from build123d import *

# Parameters (mm, degrees)
F0_R     = 4.5
F1_DEPTH = 7.5


with BuildPart() as f1:
    # F0 (on Front) → F1 (new body, symmetric)
    with BuildSketch(Plane.XZ):
        with BuildLine():
            ThreePointArc((-29.920215, -2.18649), (1.093972, -29.980047), (30, 0))
            ThreePointArc((30, 0), (21.430167, 20.993997), (0.616805, 29.993659))
            ThreePointArc((0.616805, 29.993659), (-1.441951, 29.965326), (-3.493914, 29.795848))
            ThreePointArc((-3.493914, 29.795848), (-11.688943, 27.629126), (-18.950763, 23.256582))
            ThreePointArc((-18.950763, 23.256582), (-21.461585, 20.961879), (-23.696509, 18.397703))
            ThreePointArc((-23.696509, 18.397703), (-27.765689, 11.360745), (-29.796343, 3.489695))
            ThreePointArc((-29.796343, 3.489695), (-29.992859, 0.654539), (-29.920215, -2.18649))
        make_face()
        with BuildLine():
            ThreePointArc((-8.455649, -19.222435), (-12.662502, -16.752941), (-16.186097, -13.379472))
            Line((-16.186097, -13.379472), (-5.435969, -7.172883))
            Line((-5.435969, -7.172883), (-8.455649, -19.222435))
        make_face(mode=Mode.SUBTRACT)
        with BuildLine():
            Line((-20.885863, -2.18649), (-8.730364, -2.18649))
            Line((-8.730364, -2.18649), (-18.847223, -9.261867))
            ThreePointArc((-18.847223, -9.261867), (-20.179068, -5.814227), (-20.885863, -2.18649))
        make_face(mode=Mode.SUBTRACT)
        with BuildLine():
            Line((-1.8781, -20.915849), (1.125788, -8.929311))
            Line((1.125788, -8.929311), (7.331845, -19.678517))
            ThreePointArc((7.331845, -19.678517), (2.796173, -20.813011), (-1.8781, -20.915849))
        make_face(mode=Mode.SUBTRACT)
        with BuildLine():
            Line((12.336487, -16.994443), (6.258738, -6.467473))
            Line((6.258738, -6.467473), (17.444624, -11.69124))
            ThreePointArc((17.444624, -11.69124), (15.124802, -14.568472), (12.336487, -16.994443))
        make_face(mode=Mode.SUBTRACT)
        with BuildLine():
            ThreePointArc((20.874941, 2.288411), (20.839724, -2.589578), (19.680011, -7.327835))
            Line((19.680011, -7.327835), (8.929883, -1.121246))
            Line((8.929883, -1.121246), (20.874941, 2.288411))
        make_face(mode=Mode.SUBTRACT)
        with BuildLine():
            Line((-17.174607, 12.084407), (-8.295904, 3.489695))
            Line((-8.295904, 3.489695), (-20.708019, 3.489695))
            ThreePointArc((-20.708019, 3.489695), (-19.422682, 7.984949), (-17.174607, 12.084407))
        make_face(mode=Mode.SUBTRACT)
        with BuildLine():
            ThreePointArc((-12.419293, 16.934024), (-8.177222, 19.342519), (-3.493914, 20.707307))
            Line((-3.493914, 20.707307), (-3.493914, 8.294128))
            Line((-3.493914, 8.294128), (-12.419293, 16.934024))
        make_face(mode=Mode.SUBTRACT)
        Circle(F0_R, mode=Mode.SUBTRACT)
        with BuildLine():
            Line((2.471627, 8.653962), (1.402599, 20.953108))
            ThreePointArc((1.402599, 20.953108), (5.054266, 20.382699), (8.549376, 19.180933))
            Line((8.549376, 19.180933), (2.471627, 8.653962))
        make_face(mode=Mode.SUBTRACT)
        with BuildLine():
            Line((19.052707, 8.831442), (7.170116, 5.439617))
            Line((7.170116, 5.439617), (13.376173, 16.188823))
            ThreePointArc((13.376173, 16.188823), (16.62651, 12.828062), (19.052707, 8.831442))
        make_face(mode=Mode.SUBTRACT)
    extrude(amount=F1_DEPTH, both=True)


solid = f1.part
Input: part model. Units: mm. Frame: model coordinates. Round coordinates to 2 decimals unless told otherwise and drop trailing zeros. Order: outer loops, then holes, each group sorted by start corner. A loop starts at its lowest first (then second) coordinate and runs counter-clockwise, first axis right, second up.
1. Cut plane D-D, the plane z = -25. Output: boundary loops of the cut face in (x, y).
The answers:
outline: (-16.58, -7.5) - (16.58, -7.5) - (16.58, 7.5) - (-16.58, 7.5) - close
2. Cut plane B-B, the plane y = -3. State how many separate pieces and enclosed holes the cut face has, then the cut area to 3 significant figures.
The answers:
separate pieces: 1
enclosed holes: 10
area: 2,280 mm2
3. Pin query (flat end, axial travel): P1, Ø2, axis at x = -8.5, z = 15, coming from the +Y side; P2, Ø4, axis at x = -7.5, y = 0, coming from the -Z side; P3, Ø2, axis at y = -1.5, z = -14.5, coming from the -X side. Return the tip coordinate at first contact, or that it passes through.
The answers:
P1: passes through
P2: stops at z = -29.49
P3: stops at x = -26.79
4. Mould query, pull axis X, two halves, no side actions, for faces 1 (the face through (-11.579, -0.105, 27.675)), 2 (the face through (-0.59, 0.11, 4.46)), 3 (the face through (0, 7.5, -6)). Classes: released by +X, released by -X, zero draft, split by the parting line, or undercut.
The answers:
face 1: released by -X
face 2: undercut
face 3: zero draft
5. Cut plane A-A, the plane x = 11. Output: boundary loops of the cut face in (y, z), then the cut area to 3 significant figures.
The answers:
outline: (-7.5, -27.91) - (7.5, -27.91) - (7.5, -14.68) - (-7.5, -14.68) - close; (-7.5, -8.68) - (7.5, -8.68) - (7.5, -2.32) - (-7.5, -2.32) - close; (-7.5, -0.53) - (7.5, -0.53) - (7.5, 6.53) - (-7.5, 6.53) - close; (-7.5, 12.07) - (7.5, 12.07) - (7.5, 27.91) - (-7.5, 27.91) - close
area: 637 mm2
6. Cut plane C-C, the plane x = -11. Output: boundary loops of the cut face in (y, z).
The answers:
outline: (-7.5, -27.91) - (7.5, -27.91) - (7.5, -17.89) - (-7.5, -17.89) - close; (-7.5, -10.39) - (7.5, -10.39) - (7.5, -3.77) - (-7.5, -3.77) - close; (-7.5, -2.19) - (7.5, -2.19) - (7.5, 3.49) - (-7.5, 3.49) - close; (-7.5, 6.11) - (7.5, 6.11) - (7.5, 15.56) - (-7.5, 15.56) - close; (-7.5, 17.89) - (7.5, 17.89) - (7.5, 27.91) - (-7.5, 27.91) - close
7. Material intervals for line 1 (X direction, y = -0.75, z = -8); line 2 (Z direction, x = 6, y = 3.75); line 3 (X direction, y = -5.25, z = -12), sorted ascending.
The answers:
line 1: x = -28.91 to -19.42, -17.04 to -6.87, -5.64 to 7.14, 9.54 to 28.91
line 2: z = -29.39 to -20.12, -17.37 to 14.77, 20.12 to 29.39
line 3: x = -27.5 to -13.8, -6.65 to 0.36, 2.9 to 9.45, 17.23 to 27.5
